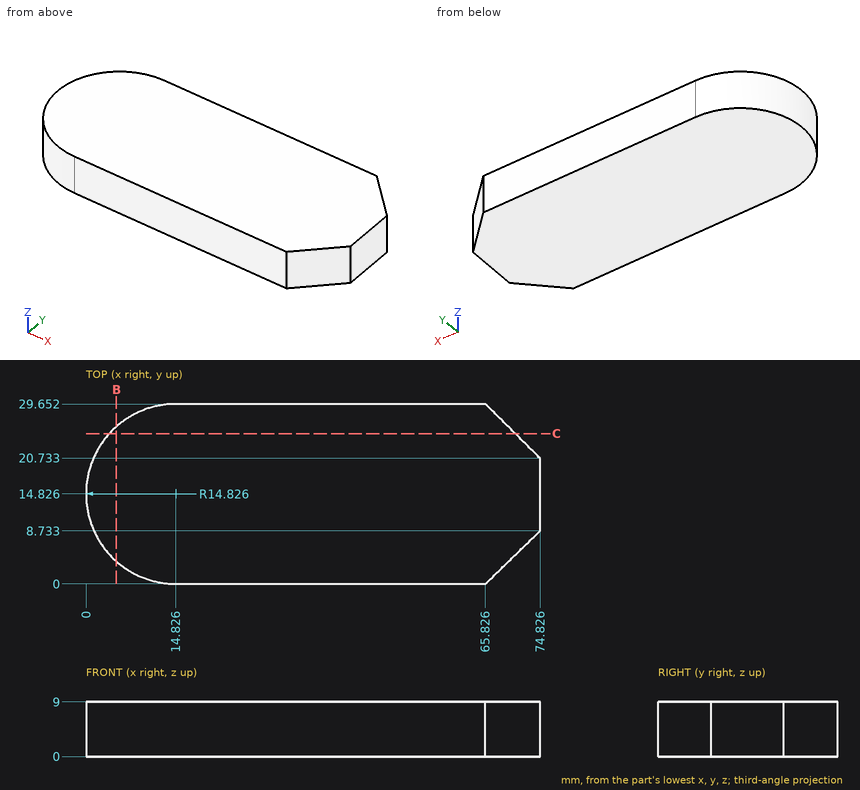
For this review, use the dimensioned drawing (mm, ordinates from the lowest corner) and the shaded views. Round coordinates to 2 decimals unless told otherwise and drop trailing zeros. Write each loop counter-clockwise with the first axis right and the second up, starting at its lowest first coordinate (ties: lowest second). Pieces come first, ordered by that corner, then holes. Notation, with made-up numbers: M 83.25,83.25 L 111.25,83.25 A36 ccw 111.25,118.25 Z; hole C -34.75,55.25 d5. An arc over 180 degrees is marked long. Answer as CSV lines item,"result". Start each with the question number.
Q1. Consider section C-C, the plane y = 24.75. Give the boundary of the cut face in (x, z).
Q2. Clearance check with flat-ended pins moving along their axes: P1, Ø10, axis at x = 59.5, y = 10, coming from the -Z side; P2, Ø5, axis at y = 3.5, z = 4.5, coming from the -X side; P3, Ø2, axis at y = 24.5, z = 3, coming from the -X side. State where each tip first meets the part, or that it passes through.
Q3. Wall thickness on line 1 along X through (y, z) = (2, 8) (1 decimal); line 2 along Y through (x, z) = (67.5, 4.5) (1 decimal); line 3 along X through (y, z) = (5.25, 2.5) (1 decimal): over which ranges is each line inside the solid? List them lowest first.
Q4. Consider section B-B, the plane x = 5. Give the boundary of the cut face in (y, z), then the cut area to 3 significant figures.
Result set:
1,outline,"M 3.81,0 L 70.77,0 L 70.77,9 L 3.81,9 Z"
2,P1,"stops at z = 0"
2,P2,"stops at x = 2.91"
2,P3,"stops at x = 2.8"
3,line 1,"x = 7.4 to 67.9"
3,line 2,"y = 1.6 to 28"
3,line 3,"x = 3.5 to 71.2"
4,outline,"M 3.72,0 L 25.93,0 L 25.93,9 L 3.72,9 Z"
4,area,"200 mm²"
